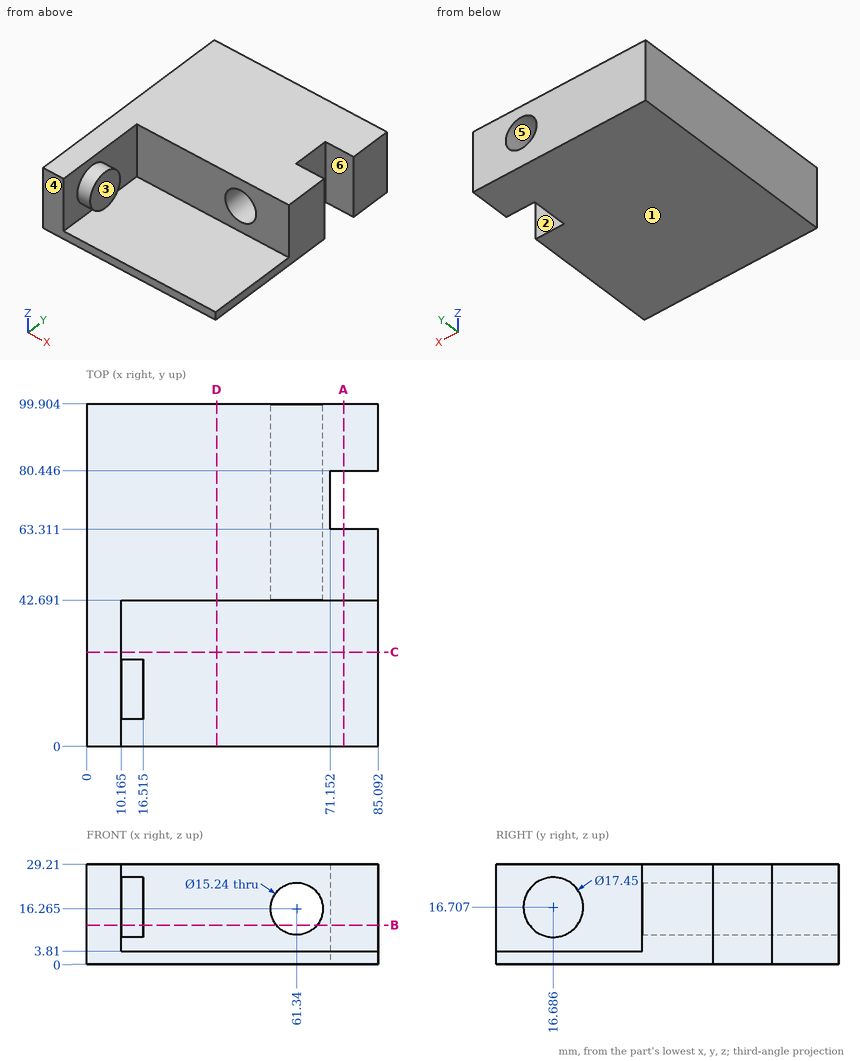
Print and shaded views of the part. All mm, measured from the part's lowest x, y and z. A direction names the side the tool comes from. Coordinates: 2 decimals unless noted, no trailing zeros. Order: outer loops, then holes, each group sorted by start corner. A loop starts at its lowest first (then second) coordinate and runs counter-clockwise, first axis right, second up. Notation, with made-up numbers: M 55.5,6.5 L 78.5,6.5 A32 ccw 78.5,44.5 Z; hole C -33,61 d5. An arc over 180 degrees is marked long. One line per question, with ' | ' between items. Start each with the question number.
Q1. 3-axis set-ups, long thin cutter, end or side, ignore diameter. For the marked faces 1, 2 and 3: which of +Z, -Z, +X, -X, +Y, -Y reach the whole face in a straight line?
Q2. Flat gauge pins, fed straight in: pin 1 Ø1 at (y, z) = (56, 12) entering from -X; pin 2 Ø7.5 at (x, z) = (63, 22) entering from -Y; pin 3 Ø4 at (x, z) = (16.5, 8.5) entering from -Y (1 decimal); pin 4 Ø2 at (x, z) = (64, 21.5) entering from -Y. Where does each tip first touch, or does it go through?
Q3. Saw through at D-D (x = 38). List the corners of the cut face in (y, z).
Q4. Two-plate mould, pull along Y, no slides. Class the marked faces 4, 5 and 6: +Y half, -Y half, draft (parallel to the pull), parting line (faces both ways), or undercut.
Q5. Probe L1, parallel to Y at x = 77, z = 23.25 (1 decimal); L2, parallel to Z at x = 40, y = 31; L3, parallel to X at y = 92, z = 16 (1 decimal). List the from-to ranges inside material, lowest first. Write a range as from..to.
Q6. Saw through at B-B (z = 11.5). List the corners of the cut face in (x, y) (1 decimal), then the cut area to 3 significant figures.
Q7. Saw through at A-A (x = 75). List the corners of the cut face in (y, z) (1 decimal).
Q8. Saw through at C-C (y = 27.5). List the corners of the cut face in (x, z) (1 decimal).
Check values:
1) face 1: -Z, +X, -X, +Y, -Y | face 2: +Z, -Z, +X | face 3: +Z, +X, -Y
2) pin 1: stops at x = 0 | pin 2: stops at y = 42.69 | pin 3: stops at y = 10.6 | pin 4: passes through
3) outline: M 0,0 L 99.9,0 L 99.9,29.21 L 42.69,29.21 L 42.69,3.81 L 0,3.81 Z
4) face 4: -Y half | face 5: draft | face 6: undercut
5) L1: y = 42.7..63.3, 80.4..99.9 | L2: z = 0..3.81 | L3: x = 0..53.7, 69..85.1
6) outline: M 0,0 L 10.2,0 L 10.2,9.7 L 16.5,9.7 L 16.5,23.7 L 10.2,23.7 L 10.2,42.7 L 55.4,42.7 L 55.4,99.9 L 0,99.9 Z; M 67.3,42.7 L 85.1,42.7 L 85.1,63.3 L 71.2,63.3 L 71.2,80.4 L 85.1,80.4 L 85.1,99.9 L 67.3,99.9 Z | area: 4,470 mm2
7) outline: M 0,0 L 63.3,0 L 63.3,29.2 L 42.7,29.2 L 42.7,3.8 L 0,3.8 Z; M 80.4,0 L 99.9,0 L 99.9,29.2 L 80.4,29.2 Z
8) outline: M 0,0 L 85.1,0 L 85.1,3.8 L 10.2,3.8 L 10.2,29.2 L 0,29.2 Z
